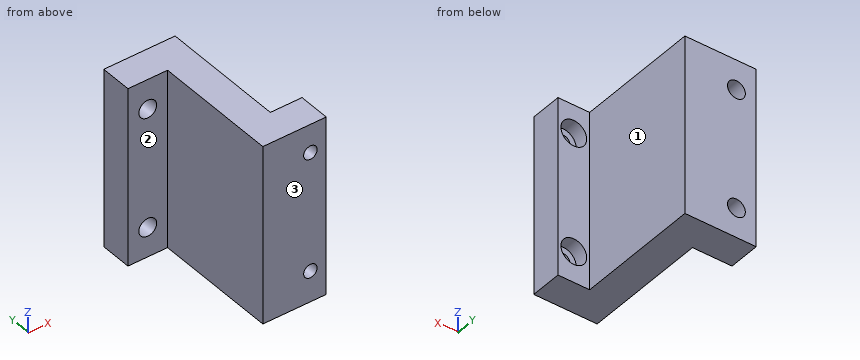
from build123d import *

# Parameters (mm, degrees)
BOSS_EXTRUDE1_DEPTH = 45
SKETCH2_R           = 2.25
CUT_EXTRUDE1_DEPTH  = 45
SKETCH3_R           = 1.7
CUT_EXTRUDE2_DEPTH  = 45
SKETCH4_R           = 3.25
CUT_EXTRUDE3_DEPTH  = 3.5


with BuildPart() as part:
    # Sketch1 → Boss-Extrude1 (new body)
    with BuildSketch(Plane.XY):
        Polygon((-4.588607595, 8.541139241), (13.411392405, 8.541139241), (13.411392405, -22.958860759), (21.411392405, -22.958860759), (21.411392405, -30.958860759), (5.411392405, -30.958860759), (5.411392405, 0.541139241), (-4.588607595, 0.541139241), align=None)
    extrude(amount=BOSS_EXTRUDE1_DEPTH)

    # Sketch2 → Cut-Extrude1 (cut)
    with BuildSketch(Plane(origin=(0, 8.541139241, 0), x_dir=(1, 0, 0), z_dir=(0, 1, 0))):
        with Locations((0.411392405, -7.5)):
            Circle(SKETCH2_R)
        with Locations((0.411392405, -37.5)):
            Circle(SKETCH2_R)
    extrude(amount=-CUT_EXTRUDE1_DEPTH, mode=Mode.SUBTRACT)

    # Sketch3 → Cut-Extrude2 (cut)
    with BuildSketch(Plane(origin=(0, -22.958860759, 0), x_dir=(1, 0, 0), z_dir=(0, 1, 0))):
        with Locations((17.411392405, -7.810599517)):
            Circle(SKETCH3_R)
        with Locations((17.411392405, -37.843221269)):
            Circle(SKETCH3_R)
    extrude(amount=-CUT_EXTRUDE2_DEPTH, mode=Mode.SUBTRACT)

    # Sketch4 → Cut-Extrude3 (cut)
    with BuildSketch(Plane(origin=(0, -22.958860759, 0), x_dir=(1, 0, 0), z_dir=(0, 1, 0))):
        with Locations((17.411392405, -7.810599517)):
            Circle(SKETCH4_R)
        with Locations((17.411392405, -37.843221269)):
            Circle(SKETCH4_R)
    extrude(amount=-CUT_EXTRUDE3_DEPTH, mode=Mode.SUBTRACT)


solid = part.part
Check sheet for the modelled part. Datum: model origin and axes. Units: mm. Face numbers are marked on the shaded views. A direction names the side the tool comes from. Round coordinates to 2 decimals unless told otherwise and drop trailing zeros. Write each loop counter-clockwise with the first axis right and the second up, starting at its lowest first coordinate (ties: lowest second). Pieces come first, ordered by that corner, then holes. Notation, with made-up numbers: (35, 54.25) -> (72, 54.25) arc R17 ccw to (72, 86.25) -> close; hole circle Ø1 at (61, 2.25). An arc over 180 degrees is marked (long way). Answer as CSV lines item,"result". Start each with the question number.
1) Section check A-A on z = 15. Enter the section's corners in (x, y).
2) Section check B-B on y = -13. Enter the section's corners in (x, z), and give its area (3 significant figures).
3) Material ranges on line 1 (Z direction, x = 17, y = -29); line 2 (Z direction, x = 16.25, y = -23); line 3 (Y direction, x = -1, z = 32), recorded low to high. Write a range as from..to.
4) Go/stop test with flat-tipped pins: P1, Ø10, axis at x = 12.5, y = -4.5, coming from the -Z side; P2, Ø6, axis at y = -17, z = 24.5, coming from the -X side; P3, Ø3, axis at x = 18, z = 29, coming from the +Y side; P4, Ø9.5, axis at y = -11, z = 22, coming from the +X side. Record where each tip stops, or that it passes through.
5) Tool access check on the marked faces 1, 2 and 3. Record the directions out of +Z, -Z, +X, -X, +Y, -Y that give a thin tool (end or side, any length) a straight path to the whole face; none if there is none.
Found:
1,outline,"(-4.59, 0.54) -> (5.41, 0.54) -> (5.41, -30.96) -> (21.41, -30.96) -> (21.41, -22.96) -> (13.41, -22.96) -> (13.41, 8.54) -> (-4.59, 8.54) -> close"
2,outline,"(5.41, 0) -> (13.41, 0) -> (13.41, 45) -> (5.41, 45) -> close"
2,area,"360 mm^2"
3,line 1,"z = 0..6.16, 9.46..36.19, 39.49..45"
3,line 2,"z = 0..4.78, 10.85..34.81, 40.88..45"
3,line 3,"y = 0.54..8.54"
4,P1,"stops at z = 0"
4,P2,"stops at x = 5.41"
4,P3,"stops at y = -22.96"
4,P4,"stops at x = 13.41"
5,face 1,"+Z, -Z, +X, +Y"
5,face 2,"+Z, -Z, -X, -Y"
5,face 3,"+Z, -Z, +X, -X, -Y"
